For this review, take the finished solid that the model builds, in its own axes (mm). A direction names the side the tool comes from. Coordinates: 2 decimals unless noted, no trailing zeros. Write each loop counter-clockwise with the first axis right and the second up, starting at its lowest first coordinate (ties: lowest second). Pieces come first, ordered by that corner, then holes.
```python
from build123d import *

# Parameters (mm, degrees)
BOSS_EXTRUDE2_DEPTH = 5
CUT_EXTRUDE5_DEPTH  = 2.5
SKETCH8_R           = 0.9
CUT_EXTRUDE6_DEPTH  = 33.308147585


with BuildPart() as part:
    # Sketch1 → Boss-Extrude2 (new body)
    with BuildSketch(Plane.XY):
        with BuildLine():
            Line((-23.25, 4.75), (-23.25, -4.75))
            Line((-23.25, -4.75), (-11.691342951, -4.75))
            ThreePointArc((-11.691342951, -4.75), (-9.949887623, -5.766468943), (-9.978567551, -7.78266666))
            Line((-9.978567551, -7.78266666), (-15.863620668, -17.543584287))
            Line((-15.863620668, -17.543584287), (-7.636379332, -22.293584287))
            Line((-7.636379332, -22.293584287), (-1.857050808, -12.283493649))
            ThreePointArc((-1.857050808, -12.283493649), (-0.106035217, -11.283583567), (1.625703261, -12.316519972))
            Line((1.625703261, -12.316519972), (7.136379332, -22.293584287))
            Line((7.136379332, -22.293584287), (15.363620668, -17.543584287))
            Line((15.363620668, -17.543584287), (9.584292144, -7.533493649))
            ThreePointArc((9.584292144, -7.533493649), (9.593852406, -5.517114624), (11.354270812, -4.533853312))
            Line((11.354270812, -4.533853312), (22.75, -4.75))
            Line((22.75, -4.75), (22.75, 4.75))
            Line((22.75, 4.75), (11.354270812, 4.533853312))
            ThreePointArc((11.354270812, 4.533853312), (9.593852406, 5.517114624), (9.584292144, 7.533493649))
            Line((9.584292144, 7.533493649), (15.363620668, 17.543584287))
            Line((15.363620668, 17.543584287), (7.136379332, 22.293584287))
            Line((7.136379332, 22.293584287), (1.625703261, 12.316519972))
            ThreePointArc((1.625703261, 12.316519972), (-0.106035217, 11.283583567), (-1.857050808, 12.283493649))
            Line((-1.857050808, 12.283493649), (-7.636379332, 22.293584287))
            Line((-7.636379332, 22.293584287), (-15.863620668, 17.543584287))
            Line((-15.863620668, 17.543584287), (-9.978567551, 7.78266666))
            ThreePointArc((-9.978567551, 7.78266666), (-9.949887623, 5.766468943), (-11.691342951, 4.75))
            Line((-11.691342951, 4.75), (-23.25, 4.75))
        make_face()
    extrude(amount=BOSS_EXTRUDE2_DEPTH)

    # Sketch7 → Cut-Extrude5 (cut)
    with BuildSketch(Plane(origin=(0, 0, 0), x_dir=(-1, 0, 0), z_dir=(0, 0, -1))):
        with BuildLine():
            Line((-6.859008781, 3.960050566), (-9.849329973, 11.622556693))
            ThreePointArc((-9.849329973, 11.622556693), (-8.6625, 15.003890121), (-5.140764367, 14.341048313))
            Line((-5.140764367, 14.341048313), (0, 7.920101132))
            Line((0, 7.920101132), (5.140764367, 14.341048313))
            ThreePointArc((5.140764367, 14.341048313), (8.6625, 15.003890121), (9.849329973, 11.622556693))
            Line((9.849329973, 11.622556693), (6.859008781, 3.960050566))
            Line((6.859008781, 3.960050566), (14.99009434, 2.71849162))
            ThreePointArc((14.99009434, 2.71849162), (17.325, 0), (14.99009434, -2.71849162))
            Line((14.99009434, -2.71849162), (6.859008781, -3.960050566))
            Line((6.859008781, -3.960050566), (9.849329973, -11.622556693))
            ThreePointArc((9.849329973, -11.622556693), (8.6625, -15.003890121), (5.140764367, -14.341048313))
            Line((5.140764367, -14.341048313), (0, -7.920101132))
            Line((0, -7.920101132), (-5.140764367, -14.341048313))
            ThreePointArc((-5.140764367, -14.341048313), (-8.6625, -15.003890121), (-9.849329973, -11.622556693))
            Line((-9.849329973, -11.622556693), (-6.859008781, -3.960050566))
            Line((-6.859008781, -3.960050566), (-14.99009434, -2.71849162))
            ThreePointArc((-14.99009434, -2.71849162), (-17.325, 0), (-14.99009434, 2.71849162))
            Line((-14.99009434, 2.71849162), (-6.859008781, 3.960050566))
        make_face()
    extrude(amount=-CUT_EXTRUDE5_DEPTH, mode=Mode.SUBTRACT)

    # Sketch8 → Cut-Extrude6 (cut, through all)
    with BuildSketch(Plane(origin=(0, 0, 2.5), x_dir=(-1, 0, 0), z_dir=(0, 0, -1))):
        with Locations((7.25, 0)):
            Circle(SKETCH8_R)
        with Locations((13.5, 0)):
            Circle(SKETCH8_R)
        with Locations((6.75, -11.691342951)):
            Circle(SKETCH8_R)
        with Locations((3.625, -6.278684177)):
            Circle(SKETCH8_R)
        with Locations((-6.75, -11.691342951)):
            Circle(SKETCH8_R)
        with Locations((-3.625, -6.278684177)):
            Circle(SKETCH8_R)
        with Locations((-13.5, 0)):
            Circle(SKETCH8_R)
        with Locations((-7.25, 0)):
            Circle(SKETCH8_R)
        with Locations((-6.75, 11.691342951)):
            Circle(SKETCH8_R)
        with Locations((-3.625, 6.278684177)):
            Circle(SKETCH8_R)
        with Locations((6.75, 11.691342951)):
            Circle(SKETCH8_R)
        with Locations((3.625, 6.278684177)):
            Circle(SKETCH8_R)
    extrude(amount=-CUT_EXTRUDE6_DEPTH, mode=Mode.SUBTRACT)


solid = part.part
```
Q1. Tool access review of faces 4 (the cylindrical face through (9.58, -5.54, 2.46)), 5 (the flat face through (-4.706, 17.218, 2.465)), 6 (the flat face through (0, 0, 2.5)): name each direction out of +Z, -Z, +X, -X, +Y, -Y from which nothing blocks a thin tool from reaching the whole face with its end or side.
Ans:
face 4: +Z, -Z
face 5: +Z, -Z, +Y
face 6: -Z
Q2. Clearance check with flat-ended pins moving along their axes: pin 1 Ø2 at (x, z) = (-1, 2.5) entering from +Y; pin 2 Ø3 at (x, y) = (-7.25, 0) entering from -Z; pin 3 Ø1.5 at (x, z) = (-18.5, 3.5) entering from +Y. State where each tip first meets the part, or that it passes through.
Ans:
pin 1: stops at y = 12.53
pin 2: stops at z = 2.5
pin 3: stops at y = 4.75
Q3. For probe 1 along Y at (x, z) = (7.5, 2.95); probe 2 along Y at (x, z) = (13, 2.45); probe 3 along X at (y, z) = (9.5, 1.7), list the stretches that pass through material, from the lowest coordinate up.
Ans:
probe 1: y = -22.08 to -12.19, -11.19 to -0.86, 0.86 to 11.19, 12.19 to 22.08
probe 2: y = -18.91 to -13.45, -4.57 to -3.02, 3.02 to 4.57, 13.45 to 18.91
probe 3: x = -11.01 to -9.02, -1.26 to 1.26, 9.02 to 10.72
Q4. Draft analysis for pull direction X (two halves, no side actions). For faces 1 (the cylindrical face through (-8.1, 0.3, 3.7)), 2 (the cylindrical face through (-9.936, 5.792, 2.465)), 3 (the flat face through (12.434, 12.468, 2.465)), state which applies: +X half, -X half, draft (parallel to the pull), parting line (faces both ways), or undercut.
Ans:
face 1: undercut
face 2: -X half
face 3: +X half
Q5. Add section D-D (x = -13.5). State the section outline as (y, z) points, then the cut area to 3 significant figures.
Ans:
outline: (-18.91, 0) - (-13.62, 0) - (-13.62, 5) - (-18.91, 5) - close; (-4.75, 0) - (-2.95, 0) - (-2.95, 2.5) - (-0.9, 2.5) - (-0.9, 5) - (-4.75, 5) - close; (0.9, 2.5) - (2.95, 2.5) - (2.95, 0) - (4.75, 0) - (4.75, 5) - (0.9, 5) - close; (13.62, 0) - (18.91, 0) - (18.91, 5) - (13.62, 5) - close
area: 81.1 mm2
Q6. Add section C-C (y = -19). State the section outline as (x, z) points, then the cut area to 4 significant figures.
Ans:
outline: (-13.34, 0) - (-5.73, 0) - (-5.73, 5) - (-13.34, 5) - close; (5.32, 0) - (12.84, 0) - (12.84, 5) - (5.32, 5) - close
area: 75.65 mm2
Q7. Add section A-A (y = 0). State the section outline as (x, z) points (3 decimals).
Ans:
outline: (-23.25, 0) - (-17.325, 0) - (-17.325, 2.5) - (-14.4, 2.5) - (-14.4, 5) - (-23.25, 5) - close; (-12.6, 2.5) - (-8.15, 2.5) - (-8.15, 5) - (-12.6, 5) - close; (-6.35, 2.5) - (6.35, 2.5) - (6.35, 5) - (-6.35, 5) - close; (8.15, 2.5) - (12.6, 2.5) - (12.6, 5) - (8.15, 5) - close; (14.4, 2.5) - (17.325, 2.5) - (17.325, 0) - (22.75, 0) - (22.75, 5) - (14.4, 5) - close
Q8. Add section B-B (x = 13.5). State the section outline as (y, z) points, then the cut area to 3 significant figures.
Ans:
outline: (-18.62, 0) - (-14.32, 0) - (-14.32, 5) - (-18.62, 5) - close; (-4.57, 0) - (-2.95, 0) - (-2.95, 2.5) - (-0.9, 2.5) - (-0.9, 5) - (-4.57, 5) - close; (0.9, 2.5) - (2.95, 2.5) - (2.95, 0) - (4.57, 0) - (4.57, 5) - (0.9, 5) - close; (14.32, 0) - (18.62, 0) - (18.62, 5) - (14.32, 5) - close
area: 69.6 mm2
